Design review of the part built by this model. Coordinates are the model's own, in mm. A direction names the side the tool comes from. Coordinates: 2 decimals unless noted, no trailing zeros. Write each loop counter-clockwise with the first axis right and the second up, starting at its lowest first coordinate (ties: lowest second). Pieces come first, ordered by that corner, then holes. Notation, with made-up numbers: M -29,-8 L 6,-8 A14 ccw 6,14 Z; hole C 4,-12.75 d9. An arc over 180 degrees is marked long. One line per question, with ' | ' between items.
from build123d import *

# Parameters (mm, degrees)
SKETCH_1_R      = 1
EXTRUDE_2_DEPTH = 3


with BuildPart() as part:
    # 草图1 → 凸台-拉伸2 (new body)
    with BuildSketch(Plane.XY):
        with BuildLine():
            Line((-8.802114216, 25.014860267), (-8.802114216, 38.857938329))
            ThreePointArc((-8.802114216, 38.857938329), (-9.402114216, 39.457938329), (-10.002114216, 38.857938329))
            Line((-10.002114216, 38.857938329), (-10.002114216, 25.014860267))
            Line((-10.002114216, 25.014860267), (-11.802114216, 25.014860267))
            Line((-11.802114216, 25.014860267), (-11.802114216, 42.39491112))
            ThreePointArc((-11.802114216, 42.39491112), (-11.725840507, 42.995157842), (-11.501867444, 43.557252027))
            Line((-11.501867444, 43.557252027), (-10.707433177, 44.992386854))
            ThreePointArc((-10.707433177, 44.992386854), (-5.982884025, 47.089313582), (-2.802114216, 43.014860267))
            Line((-2.802114216, 43.014860267), (-2.802114216, 25.014860267))
            Line((-2.802114216, 25.014860267), (-8.802114216, 25.014860267))
        make_face()
        with Locations((-7.002114216, 37.014860267)):
            Circle(SKETCH_1_R, mode=Mode.SUBTRACT)
        with Locations((-7.002114216, 31.014860267)):
            Circle(SKETCH_1_R, mode=Mode.SUBTRACT)
        with BuildLine():
            Line((-8.052114216, 43.014860267), (-8.052114216, 41.312655814))
            ThreePointArc((-8.052114216, 41.312655814), (-5.002114216, 43.014860267), (-8.052114216, 44.71706472))
            Line((-8.052114216, 44.71706472), (-8.052114216, 43.014860267))
        make_face(mode=Mode.SUBTRACT)
    extrude(amount=EXTRUDE_2_DEPTH)


solid = part.part
1. Take a section at D-D (z = 0.4). Write out the cut boundary in (x, y), then the cut area to 3 significant figures.
Answer sheet:
outline: M -11.8,25.01 L -10,25.01 L -10,38.86 A0.6 cw -8.8,38.86 L -8.8,25.01 L -2.8,25.01 L -2.8,43.01 A4.2 ccw -10.71,44.99 L -11.5,43.56 A2.4 ccw -11.8,42.39 Z; hole M -8.05,41.31 A2 ccw long -8.05,44.72 Z; hole C -7,31.01 d2; hole C -7,37.01 d2 | area: 156 mm^2
2. Take a section at C-C (y = 36.5). Write out the cut boundary in (x, z).
Answer sheet:
outline: M -11.8,0 L -10,0 L -10,3 L -11.8,3 Z; M -8.8,0 L -7.86,0 L -7.86,3 L -8.8,3 Z; M -6.14,0 L -2.8,0 L -2.8,3 L -6.14,3 Z
3. Tool access review of faces 4 (the face through (-10.002, 32, 1)), 5 (the face through (-6, 25.015, 1)), 6 (the face through (-8.052, 43, 1)): name each direction out of +Z, -Z, +X, -X, +Y, -Y from which nothing blocks a thin tool from reaching the whole face with its end or side.
Answer sheet:
face 4: +Z, -Z, -Y | face 5: +Z, -Z, +X, -X, -Y | face 6: +Z, -Z
4. Take a section at B-B (x = -7.5). Write out the cut boundary in (y, z), then the cut area to 3 significant figures.
Answer sheet:
outline: M 25.01,0 L 30.15,0 L 30.15,3 L 25.01,3 Z; M 31.88,0 L 36.15,0 L 36.15,3 L 31.88,3 Z; M 37.88,0 L 41.08,0 L 41.08,3 L 37.88,3 Z; M 44.95,0 L 47.19,0 L 47.19,3 L 44.95,3 Z | area: 44.5 mm^2
5. Draft analysis for pull direction X (two halves, no side actions). For faces 1 (the face through (-11, 25.015, 1)), 2 (the face through (-2.802, 34, 1)), 3 (the face through (-8.802, 32, 1)), state which applies: pulls with the +X half, pulls with the -X half, needs draft (parallel to the pull), parting line crosses it, or undercut.
Answer sheet:
face 1: needs draft | face 2: pulls with the +X half | face 3: undercut
6. Take a section at A-A (y = 42.75). Write out the cut boundary in (x, z), then the cut area to 3 significant figures.
Answer sheet:
outline: M -11.78,0 L -8.05,0 L -8.05,3 L -11.78,3 Z; M -5.02,0 L -2.8,0 L -2.8,3 L -5.02,3 Z | area: 17.8 mm^2
7. Insertion check: pin 1 Ø3 at (x, y) = (-7, 43.01) entering from -Z. The pin has a flat end and moves straight along its axis. Give the tip position at first contact, or say it passes through.
Answer sheet:
pin 1: z = 0
8. To check wall thickness, follow line 1 along X through (y, z) = (31, 0.4); line 2 along Y through (x, z) = (-6.25, 1.2); line 3 along X through (y, z) = (27.5, 1). State the ranges of each line that lie inside material, in increasing order. Write a range as [from, to].
Answer sheet:
line 1: [-11.8, -10], [-8.8, -8], [-6, -2.8] | line 2: [25.01, 30.36], [31.67, 36.36], [37.67, 41.16], [44.87, 47.15] | line 3: [-11.8, -10], [-8.8, -2.8]
